from build123d import *

# Parameters (mm, degrees)
BOSS_EXTRUDE1_DEPTH = 10
SKETCH2_W           = 5
SKETCH2_H           = 1
CUT_EXTRUDE1_DEPTH  = 2
SKETCH3_R           = 1.6
BOSS_EXTRUDE2_DEPTH = 10


# Read off the part's stored shape, not the designer's step: M3 Machine Threads Stud1
with BuildPart() as part:
    # Sketch1 → Boss-Extrude1 (new body)
    with BuildSketch(Plane(origin=(0, 0, 0), x_dir=(1, 0, 0), z_dir=(0, 1, 0))):
        with BuildLine():
            Line((-1.341640786, 1.2), (1.341640786, 1.2))
            ThreePointArc((1.341640786, 1.2), (0, -1.8), (-1.341640786, 1.2))
        make_face()
    extrude(amount=BOSS_EXTRUDE1_DEPTH)

    # Sketch2 → Cut-Extrude1 (cut)
    with BuildSketch(Plane(origin=(0, 10, 0), x_dir=(1, 0, 0), z_dir=(0, 1, 0))):
        Rectangle(SKETCH2_W, SKETCH2_H)
    extrude(amount=-CUT_EXTRUDE1_DEPTH, mode=Mode.SUBTRACT)

    # Sketch3 → Boss-Extrude2 (add)
    with BuildSketch(Plane.XZ):
        with Locations(Location((0, 0, 0), (0, 0, 228.590377891))):
            Circle(SKETCH3_R)
    extrude(amount=BOSS_EXTRUDE2_DEPTH)

    # M3 Machine Threads Stud1 outline → M3 Machine Threads Stud1 (revolve, cut)
    with BuildSketch(Plane.XY):
        Polygon((1.6, 0), (1.5, 0), (1.5, -9.7195), (1.2195, -10), (1.6, -10), align=None)
    revolve(axis=Axis((0, 0, 0), (0, 1, 0)), mode=Mode.SUBTRACT)


solid = part.part
Can you work these out from the model? Positions are in its coordinate system, mm. A direction names the side the tool comes from. Give positions to 0.01 mm unless a question says otherwise; leave off trailing zeros. Order: outer loops, then holes, each group sorted by start corner. A loop starts at its lowest first (then second) coordinate and runs counter-clockwise, first axis right, second up. Notation, with made-up numbers: M 32,-8 L 61,-8 A13 cw 61,11 Z; hole C -13.75,-11.5 d4. An arc over 180 degrees is marked long. One line per question, with ' | ' between items.
Item 1: I'm going to push a flat-ended pin straight in: pin 1 Ø2 at (x, y) = (-1, 9) entering from -Z. Where does the tip first touch, or does it pass through?
Answer block:
pin 1: stops at z = -1.2
Item 2: Suppose I cut it at D-D, the plane y = -2.25. Write out the boundary of the cut face in (x, z).
Answer block:
outline: C 0,0 d3
Item 3: Suppose I cut it at A-A, the plane z = 0. Write out the boundary of the cut face in (x, y).
Answer block:
outline: M -1.8,0 L -1.5,0 L -1.5,-9.72 L -1.22,-10 L 1.22,-10 L 1.5,-9.72 L 1.5,0 L 1.8,0 L 1.8,8 L -1.8,8 Z
Item 4: Please list where these lines run through material, in increasing order: L1, parallel to Z at x = -0.1, y = 5.5; L2, parallel to Y at x = 0.35, z = 0.45; L3, parallel to Z at x = 1.45, y = 8.5.
Answer block:
L1: z = -1.2 to 1.8 | L2: y = -10 to 8 | L3: z = -1.07 to -0.5, 0.5 to 1.07
Item 5: We'd pull the mould along Z, two halves only. Please class faces 1 (the face through (0, -10, 0)), 2 (the face through (-1.5, -4.93, -0.07)), 3 (the face through (0, 5, -1.2)), 4 (the face through (0, 8, 0)): released by +Z, released by -Z, zero draft, split by the parting line, or undercut.
Answer block:
face 1: zero draft | face 2: split by the parting line | face 3: released by -Z | face 4: undercut
Item 6: Suppose I cut it at B-B, the plane x = 0. Write out the boundary of the cut face in (y, z).
Answer block:
outline: M -10,-1.22 L -9.72,-1.5 L 0,-1.5 L 0,-1.2 L 10,-1.2 L 10,-0.5 L 8,-0.5 L 8,0.5 L 10,0.5 L 10,1.8 L 0,1.8 L 0,1.5 L -9.72,1.5 L -10,1.22 Z
Item 7: For faces 5 (the face through (0, 9, 0.5)), 6 (the face through (0.06, 4.93, 1.8)), which set-ups out of +Z, -Z, +X, -X, +Y, -Y let a thin tool reach every point of the face, with its end or its side?
Answer block:
face 5: +X, -X, +Y | face 6: +Y, -Y
Item 8: Suppose I cut it at C-C, the plane y = 0.25. Write out the boundary of the cut face in (x, z).
Answer block:
outline: M -1.34,-1.2 L 1.34,-1.2 A1.8 ccw long Z
